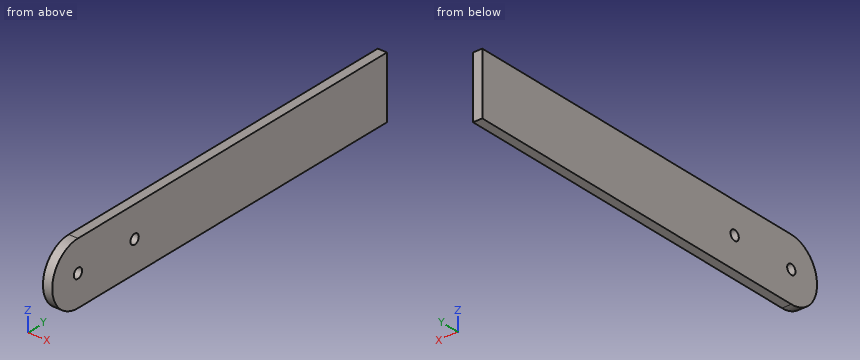
Autodesk Inventor part; units mm, degrees
ref_plane "YZ Plane" through (0, 0, 0) normal (1, 0, 0) x (0, 1, 0)
ref_plane "XZ Plane" through (0, 0, 0) normal (0, 1, 0) x (-1, 0, 0)
ref_plane "XY Plane" through (0, 0, 0) normal (0, 0, 1) x (1, 0, 0)
sketch "Szkic1" plane through (0, 0, 0) normal (1, 0, 0) x (0, 1, 0)
  line L0 (10, 0) -> (130, 0)
  line L1 (130, 0) -> (130, 20)
  line L2 (130, 20) -> (10, 20)
  line L3 (0, 10) -> (0, 10)
  arc A0 (0, 10) -> (10, 0) centre (10, 10) ccw
  arc A1 (10, 20) -> (0, 10) centre (10, 10) ccw
  circle A2 centre (32, 10) radius 1.6
  point P0 (0, 0)
  point P1 (0, 20)
  dimension "d0" = 20
  dimension "d2" = 10
  dimension "d12" = 120
  dimension "d13" = 32
  dimension "d14" = 3.2
extrude "Wyciągnięcie proste1" add sketch "Szkic1" along normal blind 3 contours A0 A1 L2 L1 L0 | A2
sketch "Szkic2" plane through (3, 0, 0) normal (1, 0, 0) x (0, 0, -1)
  arc A0 (-20, 10) -> (0, 10) centre (-10, 10) ccw
  point P0 (0, 0)
hole "Otwór1" at (3, 10, 10) direction (-1, 0, 0) diameter 3.2 end through all
sketch "Szkic3" plane through (3, 0, 0) normal (1, 0, 0) x (0, 0, -1)
  point P0 (0, 0)
  point P1 (-10, 32)
  dimension "d15" = 32
hole "Otwór2" at (3, 32, 10) direction (-1, 0, 0) diameter 3.2 end through all
properties material "Drewno (wiśnia)"
Work out the finished part from the listing and answer in its coordinate system (mm). Round coordinates to 2 decimals unless told otherwise and drop trailing zeros. Order: outer loops, then holes, each group sorted by start corner. A loop starts at its lowest first (then second) coordinate and runs counter-clockwise, first axis right, second up. Notation, with made-up numbers: M 29,74 L 52,74 A17 ccw 52,81 Z; hole C 13,28 d10. An arc over 180 degrees is marked long. One line per item, written item: value.
Q1. Find section A-A on z = 10. Write down the section's boundary in (x, y), then the cut area to 3 significant figures.
Derived:
outline: M 0,0 L 3,0 L 3,8.4 L 0,8.4 Z; M 0,11.6 L 3,11.6 L 3,30.4 L 0,30.4 Z; M 0,33.6 L 3,33.6 L 3,130 L 0,130 Z
area: 371 mm²
Q2. Find section C-C on x = 2. Write down the section's boundary in (y, z).
Derived:
outline: M 10,0 L 130,0 L 130,20 L 10,20 A10 ccw Z; hole C 10,10 d3.2; hole C 32,10 d3.2
Q3. Find section B-B on y = 32. Write down the section's boundary in (x, z).
Derived:
outline: M 0,0 L 3,0 L 3,8.4 L 0,8.4 Z; M 0,11.6 L 3,11.6 L 3,20 L 0,20 Z
Q4. Straight lines are drawn through the part: line 1 (Y direction, x = 2.3, z = 10); line 2 (Z direction, x = 0.85, y = 32); line 3 (Y direction, x = 2.8, z = 11). For each, find the intervals that lie inside material, in ascending order.
Derived:
line 1: 0 to 8.4, 11.6 to 30.4, 33.6 to 130
line 2: 0 to 8.4, 11.6 to 20
line 3: 0.05 to 8.75, 11.25 to 30.75, 33.25 to 130
Q5. A flat-ended cylindrical pin translates along its axis: pin 1 (1.5 mm diameter, centred on y = 58, z = 15, fed in from -X). Find the tip coordinate at first contact, or state that the pin passes through.
Derived:
pin 1: x = 0
Q6. Find section D-D on z = 2.75. Write down the section's boundary in (x, y), then the cut area to 3 significant figures.
Derived:
outline: M 0,3.11 L 3,3.11 L 3,130 L 0,130 Z
area: 381 mm²
